Autodesk Inventor part; units mm, degrees
ref_plane "YZ Plane" through (0, 0, 0) normal (1, 0, 0) x (0, 1, 0)
ref_plane "XZ Plane" through (0, 0, 0) normal (0, 1, 0) x (-1, 0, 0)
ref_plane "XY Plane" through (0, 0, 0) normal (0, 0, 1) x (1, 0, 0)
sketch "Sketch1" plane through (0, 0, 0) normal (0, 0, 1) x (1, 0, 0)
  line L0 (0, 0) -> (0, -17) construction
  line L1 (-3.4641, -6) -> (-6.9282, 0)
  line L2 (-6.9282, 0) -> (-3.4641, 6)
  line L3 (-3.4641, 6) -> (3.4641, 6)
  line L4 (3.4641, 6) -> (6.9282, 0)
  line L5 (6.9282, 0) -> (3.4641, -6)
  line L6 (3.4641, -6) -> (-3.4641, -6)
  point P0 (0, -6)
  dimension "d0" = 12
extrude "Extrusion1" add sketch "Sketch1" along normal blind 10
hole "Hole1" at (0, 0, 0) direction (0, 0, 1) diameter 4 end through all counterbore diameter 8 counterbore depth 8
thread "Thread1"
properties part number "HUDSON-1-80"
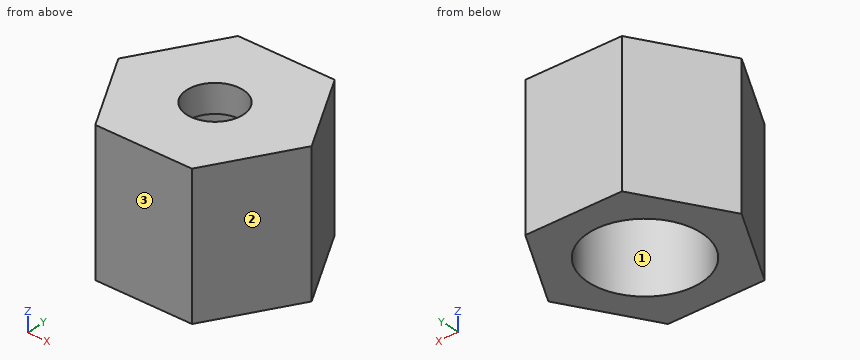
Read the model definition and answer for the solid it produces. Units are mm, in the model's axes. Face numbers are marked on the shaded views. Give positions to 0.01 mm unless a question says otherwise; leave off trailing zeros. Order: outer loops, then holes, each group sorted by start corner. A loop starts at its lowest first (then second) coordinate and runs counter-clockwise, first axis right, second up. Notation, with made-up numbers: (15.5, -23.5) -> (31.5, -23.5) arc R23 ccw to (31.5, -7.5) -> close; hole circle Ø10 at (88, 3.25). An arc over 180 degrees is marked (long way). Write item = value, one per line.
1. A cutting plane is placed at B-B, the plane y = -0.5. Write down the section's boundary in (x, z).
Numbers:
outline = (-6.64, 0) -> (-3.97, 0) -> (-3.97, 8) -> (-1.94, 8) -> (-1.94, 10) -> (-6.64, 10) -> close; (1.94, 8) -> (3.97, 8) -> (3.97, 0) -> (6.64, 0) -> (6.64, 10) -> (1.94, 10) -> close
2. A cutting plane is placed at C-C, the plane z = 7. Write down the section's boundary in (x, y).
Numbers:
outline = (-6.93, 0) -> (-3.46, -6) -> (3.46, -6) -> (6.93, 0) -> (3.46, 6) -> (-3.46, 6) -> close; hole circle Ø8 at (0, 0)
3. Straight lines are drawn through the part: line 1 along Y through (x, z) = (0, 6); line 2 along Y through (x, z) = (2, 4.5); line 3 along X through (y, z) = (2.75, 5.25). For each, find the intervals that lie inside material, in ascending order.
Numbers:
line_1 = -6 to -4, 4 to 6
line_2 = -6 to -3.46, 3.46 to 6
line_3 = -5.34 to -2.9, 2.9 to 5.34
4. A cutting plane is placed at A-A, the plane x = 0. Write down the section's boundary in (y, z).
Numbers:
outline = (-6, 0) -> (-4, 0) -> (-4, 8) -> (-2, 8) -> (-2, 10) -> (-6, 10) -> close; (2, 8) -> (4, 8) -> (4, 0) -> (6, 0) -> (6, 10) -> (2, 10) -> close
5. Given pin 1 (4 mm diameter, centred on x = 1.5, y = 0, fed in from -Z); pin 2 (5 mm diameter, centred on y = 4.5, z = 9, fed in from +X); pin 3 (4 mm diameter, centred on y = -3.5, z = 4.5, fed in from -X); pin 4 (6.5 mm diameter, centred on x = 0, y = 0, fed in from +Z), each flat-ended and moving along its own axis, determine where each tip first touches the part or whether it passes through.
Numbers:
pin_1 = 8
pin_2 = 5.77
pin_3 = -6.06
pin_4 = 10
6. The mould has two halves that part along X. Classify the marked faces 1, 2 and 3: +X half, -X half, draft (parallel to the pull), parting line (faces both ways), or undercut.
Numbers:
face_1 = undercut
face_2 = +X half
face_3 = draft
7. A cutting plane is placed at D-D, the plane y = -3.25. Write down the section's boundary in (x, z), and give its area (3 significant figures).
Numbers:
outline = (-5.05, 0) -> (-2.33, 0) -> (-2.33, 8) -> (2.33, 8) -> (2.33, 0) -> (5.05, 0) -> (5.05, 10) -> (-5.05, 10) -> close
area = 63.7 mm²
